Read the model definition and answer for the solid it produces. Units are mm, in the model's axes. A direction names the side the tool comes from. Coordinates: 2 decimals unless noted, no trailing zeros. Order: outer loops, then holes, each group sorted by start corner. A loop starts at its lowest first (then second) coordinate and runs counter-clockwise, first axis right, second up. Notation, with made-up numbers: M 26,41.25 L 55,41.25 A21 cw 55,64.25 Z; hole C 26,53 d8. An arc over 180 degrees is marked long. Put each result on its own line as item: value.
from build123d import *

# Parameters (mm, degrees)
SKETCH_1_R          = 25
EXTRUDE_1_DEPTH     = 10
SKETCH_2_R          = 10
EXTRUDE_2_DEPTH     = 10
FILLET_1_R          = 2
SKETCH_3_W          = 80
SKETCH_3_H          = 44
EXTRUDE_3_DEPTH     = 5
SKETCH_4_W          = 80
SKETCH_4_H          = 5
EXTRUDE_4_DEPTH     = 10
SKETCH_5_R          = 2
CUT_EXTRUDE_1_DEPTH = 81
FILLET_4_R          = 2


with BuildPart() as part:
    # 草圖1 → 填料-伸長1 (new body)
    with BuildSketch(Plane(origin=(0, 0, 0), x_dir=(1, 0, 0), z_dir=(0, 1, 0))):
        Circle(SKETCH_1_R)
    extrude(amount=EXTRUDE_1_DEPTH)

    # 草圖2 → 填料-伸長2 (add)
    with BuildSketch(Plane.XZ):
        Circle(SKETCH_2_R)
    extrude(amount=EXTRUDE_2_DEPTH)

    # 圓角1
    fillet_1_edges = [part.edges().sort_by_distance(p)[0] for p in [
        (-25, 0, 0),
        (-10, -10, 0),
    ]]
    fillet(fillet_1_edges, radius=FILLET_1_R)

    # 草圖3 → 填料-伸長3 (add)
    with BuildSketch(Plane(origin=(0, 10, 0), x_dir=(1, 0, 0), z_dir=(0, 1, 0))):
        Rectangle(SKETCH_3_W, SKETCH_3_H)
    extrude(amount=EXTRUDE_3_DEPTH)

    # 草圖4 → 填料-伸長4 (add)
    with BuildSketch(Plane(origin=(0, 15, 0), x_dir=(1, 0, 0), z_dir=(0, 1, 0))):
        with Locations((0, 19.5)):
            Rectangle(SKETCH_4_W, SKETCH_4_H)
        with Locations((0, -19.5)):
            Rectangle(SKETCH_4_W, SKETCH_4_H)
    extrude(amount=EXTRUDE_4_DEPTH)

    # 草圖5 → 除料-伸長1 (cut)
    with BuildSketch(Plane(origin=(0, 0, -22), x_dir=(-1, 0, 0), z_dir=(0, 0, -1))):
        with Locations((-15, 19.545082089)):
            Circle(SKETCH_5_R)
        with Locations((-35, 19.545082089)):
            Circle(SKETCH_5_R)
        with Locations((15, 19.545082089)):
            Circle(SKETCH_5_R)
        with Locations((35, 19.545082089)):
            Circle(SKETCH_5_R)
    extrude(amount=-CUT_EXTRUDE_1_DEPTH, mode=Mode.SUBTRACT)

    # 圓角4
    fillet_4_edges = [part.edges().sort_by_distance(p)[0] for p in [
        (40, 17.5, 22),
        (40, 17.5, -22),
        (-40, 17.5, -22),
        (-40, 17.5, 22),
    ]]
    fillet(fillet_4_edges, radius=FILLET_4_R)


solid = part.part
Q1. A tool of negligible diameter and unlimited length cuts with its end or side. For faces 4 (the face through (-1, 20, 17)), 5 (the face through (23.846, 5.944, -7.509)), 6 (the face through (0, 10, -23)), from which of +Z, -Z, +X, -X, +Y, -Y can it reach the whole face along a straight path? Write none if from no direction.
Answers below:
face 4: +X, -X, +Y
face 5: -Y
face 6: -Z, +X, -X, +Y
Q2. Consider line 1 along Z through (x, y) = (-20.5, 22.5); line 2 along Y through (x, z) = (-28, -14); line 3 along Y through (x, z) = (15, 20.75). Determine where each line is inside the solid, lowest interval first.
Answers below:
line 1: z = -22 to -17, 17 to 22
line 2: y = 10 to 15
line 3: y = 10 to 17.55, 21.55 to 25
Q3. For a pull along X with two mould halves and no side action, classify faces 1 (the face through (-1, 15, 0)), 2 (the face through (39.4, 17.4, -21.43)), 3 (the face through (33.092, 20.146, 19.465)) as +X half, -X half, draft (parallel to the pull), parting line (faces both ways), or undercut.
Answers below:
face 1: draft
face 2: +X half
face 3: undercut
Q4. Find section A-A on x = -35. Write down the section's boundary in (y, z).
Answers below:
outline: M 10,-22 L 17.55,-22 L 17.55,-17 L 15,-17 L 15,17 L 17.55,17 L 17.55,22 L 10,22 Z; M 21.55,-22 L 25,-22 L 25,-17 L 21.55,-17 Z; M 21.55,17 L 25,17 L 25,22 L 21.55,22 Z
Q5. Given pin 1 (5 mm diameter, centred on x = -12, y = 17, fed in from -Z); pin 2 (4.5 mm diameter, centred on x = 35, y = 19.55, fed in from +Z); pin 3 (2 mm diameter, centred on x = -29.5, z = -10, fed in from -Y), each flat-ended and moving along its own axis, determine where each tip first touches the part or whether it passes through.
Answers below:
pin 1: stops at z = -22
pin 2: stops at z = 22
pin 3: stops at y = 10
Q6. Find section C-C on y = -2. Write down the section's boundary in (x, z).
Answers below:
outline: C 0,0 d20
Q7. Find section D-D on x = 29.5. Write down the section's boundary in (y, z).
Answers below:
outline: M 10,-22 L 25,-22 L 25,-17 L 15,-17 L 15,17 L 25,17 L 25,22 L 10,22 Z
Q8. Find section B-B on z = 0. Write down the section's boundary in (x, y).
Answers below:
outline: M -40,10 L -25,10 L -25,2 A2 ccw -23,0 L -10,0 L -10,-8 A2 ccw -8,-10 L 8,-10 A2 ccw 10,-8 L 10,0 L 23,0 A2 ccw 25,2 L 25,10 L 40,10 L 40,15 L -40,15 Z
